Source: CAD feature listing. Evaluate the final solid. Frame: model axes, mm. A direction names the side the tool comes from. Round coordinates to 2 decimals unless told otherwise and drop trailing zeros. Loops run counter-clockwise (first coordinate to the right, second up) from the corner with the lowest first, then second, coordinate; pieces in that order, holes last. Notation, with made-up numbers: (64, 20) - (92, 20) arc R31 ccw to (92, 45) - close; hole circle Ø1 at (3, -18). An arc over 180 degrees is marked (long way). One line per question, with ' | ' between items. Start each with the question number.
1. Ray query, line 1 (Z direction, x = 0, y = -1.6) (3 decimals); line 2 (X direction, y = -0.25, z = -1.5); line 3 (X direction, y = -1.7, z = 3.5). Return the intervals inside material, ascending.
2. Cut plane D-D (x = 37.5). Return loops of the section in (y, z).
3. Cut plane C-C (x = 15.5). Return loops of the section in (y, z), then the cut area to 3 significant figures.
4. Mould query, pull axis Z, two halves, no side actions, for faces 3 (the cylindrical face through (21.674, -2.348, -6.675)), 4 (the flat face through (14, 0, 7)), 5 (the cylindrical face through (-0.69, -2.35, -3.1)). Classes: pulls with the +Z half, pulls with the -Z half, needs draft (parallel to the pull), parting line crosses it, or undercut.
5. Pin query (flat end, axial travel): pin 1 (2.5 mm diameter, centred on x = 1, y = -1.5, fed in from -Z). Return the tip coordinate at first contact, or that it passes through.
6. Cut plane B-B (z = 0). Return loops of the section in (x, y) (1 decimal), then the cut area to 3 significant figures.
7. Access query for faces 1 (the flat face through (1, -2, -6.241)), 2 (the flat face through (41.214, -2, 4)). Directions: +Z, -Z, +X, -X, +Y, -Y. A direction counts if a zero-diameter tool reaches every point of the face in a straight line with its end or side. Return the directions, or none.
```python
from build123d import *

# Parameters (mm, degrees)
F0_R     = 3.175
F1_DEPTH = 4.7625


with BuildPart() as f1:
    # F0 (on Front) → F1 (new body)
    with BuildSketch(Plane.XZ):
        with BuildLine():
            Line((41.21404, 16.7132), (-26.9875, 16.7132))
            Line((-26.9875, 16.7132), (-26.9875, 15.1257))
            ThreePointArc((-26.9875, 15.1257), (-26.085416, 12.83013), (-23.8125, 11.872399))
            Line((-23.8125, 11.872399), (-14.2875, 11.872399))
            ThreePointArc((-14.2875, 11.872399), (-11.24722, 10.349956), (-9.997112, 7.187936))
            Line((-9.997112, 7.187936), (-9.951094, 3.175))
            ThreePointArc((-9.951094, 3.175), (-7.123186, -3.489477), (-0.42672, -6.24078))
            Line((-0.42672, -6.24078), (2.60604, -6.24078))
            ThreePointArc((2.60604, -6.24078), (21.944184, -6.689743), (41.21404, -8.37438))
            Line((41.21404, -8.37438), (41.21404, 16.7132))
        make_face()
        Circle(F0_R, mode=Mode.SUBTRACT)
    extrude(amount=F1_DEPTH)


solid = f1.part
```
Answers follow:
1) line 1: z = -6.241 to -3.175, 3.175 to 16.713 | line 2: x = -8.66 to -2.8, 2.8 to 41.21 | line 3: x = -9.95 to 41.21
2) outline: (-4.76, -7.95) - (0, -7.95) - (0, 16.71) - (-4.76, 16.71) - close
3) outline: (-4.76, -6.4) - (0, -6.4) - (0, 16.71) - (-4.76, 16.71) - close | area: 110 mm2
4) face 3: pulls with the -Z half | face 4: needs draft | face 5: undercut
5) pin 1: stops at z = -6.24
6) outline: (-9.4, -4.8) - (-3.2, -4.8) - (-3.2, 0) - (-9.4, 0) - close; (3.2, -4.8) - (41.2, -4.8) - (41.2, 0) - (3.2, 0) - close | area: 211 mm2
7) face 1: -Z, -X, +Y, -Y | face 2: +Z, -Z, +X, +Y, -Y
